```python
from build123d import *

# Parameters (mm, degrees)
SKETCH1_R           = 1.75
SKETCH1_R_2         = 1.5
SKETCH1_R_3         = 1.7
BOSS_EXTRUDE1_DEPTH = 3


with BuildPart() as part:
    # Sketch1 → Boss-Extrude1 (new body)
    with BuildSketch(Plane.XY):
        with BuildLine():
            Line((-75, 50), (75, 50))
            ThreePointArc((75, 50), (82.071067812, 47.071067812), (85, 40))
            Line((85, 40), (85, -40))
            ThreePointArc((85, -40), (82.071067812, -47.071067812), (75, -50))
            Line((75, -50), (-75, -50))
            ThreePointArc((-75, -50), (-82.071067812, -47.071067812), (-85, -40))
            Line((-85, -40), (-85, 40))
            ThreePointArc((-85, 40), (-82.071067812, 47.071067812), (-75, 50))
        make_face()
        with Locations((-75.5, 15)):
            Circle(SKETCH1_R, mode=Mode.SUBTRACT)
        with Locations((-75.5, -15)):
            Circle(SKETCH1_R, mode=Mode.SUBTRACT)
        with Locations((-51.5, -15)):
            Circle(SKETCH1_R, mode=Mode.SUBTRACT)
        with Locations((-51.5, 15)):
            Circle(SKETCH1_R, mode=Mode.SUBTRACT)
        with Locations((75.5, -15)):
            Circle(SKETCH1_R, mode=Mode.SUBTRACT)
        with Locations((51.5, -15)):
            Circle(SKETCH1_R, mode=Mode.SUBTRACT)
        with Locations((51.5, 15)):
            Circle(SKETCH1_R, mode=Mode.SUBTRACT)
        with Locations((75.5, 15)):
            Circle(SKETCH1_R, mode=Mode.SUBTRACT)
        with Locations((-75, -40)):
            Circle(SKETCH1_R_2, mode=Mode.SUBTRACT)
        with Locations((-75, 40)):
            Circle(SKETCH1_R_2, mode=Mode.SUBTRACT)
        with Locations((75, 40)):
            Circle(SKETCH1_R_2, mode=Mode.SUBTRACT)
        with Locations((75, -40)):
            Circle(SKETCH1_R_2, mode=Mode.SUBTRACT)
        with Locations((-22.5, 25)):
            Circle(SKETCH1_R_3, mode=Mode.SUBTRACT)
        with Locations((22.5, 25)):
            Circle(SKETCH1_R_3, mode=Mode.SUBTRACT)
        with Locations((22.5, -25)):
            Circle(SKETCH1_R_3, mode=Mode.SUBTRACT)
        with Locations((-22.5, -25)):
            Circle(SKETCH1_R_3, mode=Mode.SUBTRACT)
        with BuildLine():
            Line((-25, 45), (25, 45))
            ThreePointArc((25, 45), (30, 40), (25, 35))
            Line((25, 35), (-25, 35))
            ThreePointArc((-25, 35), (-30, 40), (-25, 45))
        make_face(mode=Mode.SUBTRACT)
        with BuildLine():
            Line((-25, -45), (25, -45))
            ThreePointArc((25, -45), (30, -40), (25, -35))
            Line((25, -35), (-25, -35))
            ThreePointArc((-25, -35), (-30, -40), (-25, -45))
        make_face(mode=Mode.SUBTRACT)
    extrude(amount=BOSS_EXTRUDE1_DEPTH)


solid = part.part
```
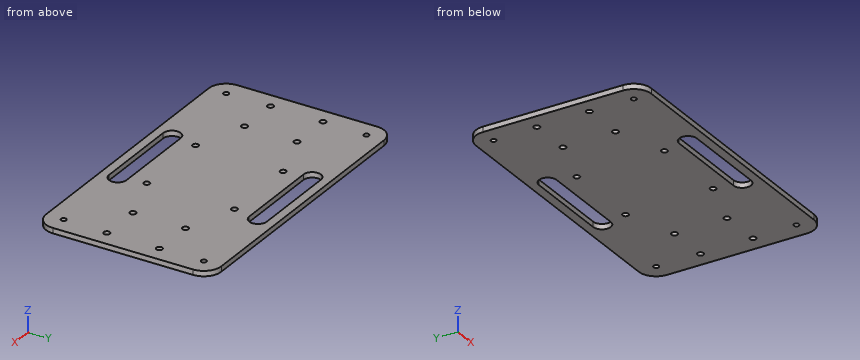
Geometry check sheet. Reference: the model listing, model coordinates, mm. Coordinates: 2 decimals unless noted, no trailing zeros. Write each loop counter-clockwise with the first axis right and the second up, starting at its lowest first coordinate (ties: lowest second). Pieces come first, ordered by that corner, then holes. Notation, with made-up numbers: M -0.75,46.5 L 46.25,46.5 A28 cw 46.25,83.5 Z; hole C 21,29.25 d5. An arc over 180 degrees is marked long. Answer as a JSON object with one key per item and string values.
1. Section check B-B, the plane x = -22.5. Enter the section's corners in (y, z), plus the area to 3 significant figures.
Answers below:
{"outline": "M -50,0 L -45,0 L -45,3 L -50,3 Z; M -35,0 L -26.7,0 L -26.7,3 L -35,3 Z; M -23.3,0 L 23.3,0 L 23.3,3 L -23.3,3 Z; M 26.7,0 L 35,0 L 35,3 L 26.7,3 Z; M 45,0 L 50,0 L 50,3 L 45,3 Z", "area": "220 mm²"}
2. Section check D-D, the plane x = 51.5. Enter the section's corners in (y, z), plus the area to 3 significant figures.
Answers below:
{"outline": "M -50,0 L -16.75,0 L -16.75,3 L -50,3 Z; M -13.25,0 L 13.25,0 L 13.25,3 L -13.25,3 Z; M 16.75,0 L 50,0 L 50,3 L 16.75,3 Z", "area": "279 mm²"}
3. Section check C-C, the plane z = 0.6. Give the number of separate pieces and of enclosed holes in the cut face, plus the area to 3 significant figures.
Answers below:
{"separate pieces": "1", "enclosed holes": "18", "area": "15,600 mm²"}
4. Scan lines: L1, parallel to Y at x = -4.5, z = 0.95; L2, parallel to Y at x = -51.5, z = 1.6; L3, parallel to Y at x = -75, z = 1.1. Record each from-to range of solid material in increasing order.
Answers below:
{"L1": "y = -50 to -45, -35 to 35, 45 to 50", "L2": "y = -50 to -16.75, -13.25 to 13.25, 16.75 to 50", "L3": "y = -50 to -41.5, -38.5 to -16.68, -13.32 to 13.32, 16.68 to 38.5, 41.5 to 50"}
5. Section check A-A, the plane y = -25. Enter the section's corners in (x, z), plus the area to 3 significant figures.
Answers below:
{"outline": "M -85,0 L -24.2,0 L -24.2,3 L -85,3 Z; M -20.8,0 L 20.8,0 L 20.8,3 L -20.8,3 Z; M 24.2,0 L 85,0 L 85,3 L 24.2,3 Z", "area": "490 mm²"}
